Check sheet for the drawn part. Datum: minimum x, y, z corner. Units: mm. A direction names the side the tool comes from. Coordinates: 2 decimals unless noted, no trailing zeros. Loops run counter-clockwise (first coordinate to the right, second up) from the corner with the lowest first, then second, coordinate; pieces in that order, holes last. Notation, with made-up numbers: (84, 4) - (118, 4) arc R8 cw to (118, 12) - close; hole circle Ø8 at (-2.75, -15). An arc over 180 degrees is marked (long way). Answer as CSV lines item,"result". Start each with the question number.
1. Material ranges on line 1 (Y direction, x = 7.5, z = 1); line 2 (X direction, y = 7, z = 1); line 3 (Z direction, x = 5.5, y = 33), recorded low to high. Write a range as [from, to].
2. Cross-section at C-C (z = 22.5). Enter the section's corners in (x, y).
3. Set-up check for the marked faces 1 and 2: record each of +Z, -Z, +X, -X, +Y, -Y from which the full face is reachable in a straight line by a thin tool's end or side.
4. Cross-section at A-A (x = 31.5). Enter the section's corners in (y, z).
5. Release check for a two-part mould opening along X. For the marked faces 3 and 4 record: pulls with the +X half, pulls with the -X half, needs draft (parallel to the pull), parting line crosses it, or undercut.
6. Gauge pin test, flat ends, axial feed: P1, Ø3, axis at y = 10.5, z = 35.5, coming from the +X side (1 decimal); P2, Ø12, axis at x = 48, z = 53.5, coming from the +Y side; P3, Ø6.5, axis at x = 7.5, y = 55.5, coming from the +Z side. Record the tip position at first contact, or that the pin passes through.
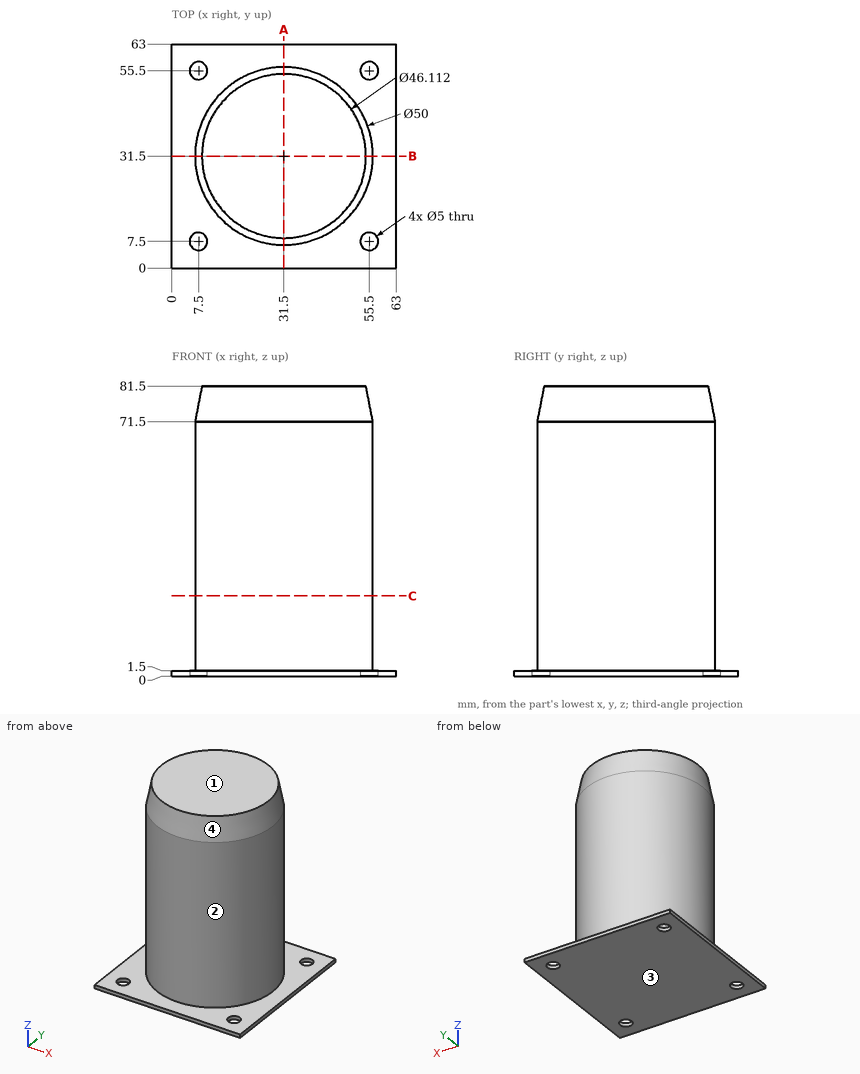
Values follow:
1,line 1,"y = [0, 5], [10, 53], [58, 63]"
1,line 2,"x = [0, 5.05], [9.95, 53.05], [57.95, 63]"
1,line 3,"z = [0, 1.5]"
2,outline,"circle Ø50 at (31.5, 31.5)"
3,face 1,"+Z, +X, -X, +Y, -Y"
3,face 2,"+Z"
4,outline,"(0, 0) - (63, 0) - (63, 1.5) - (56.5, 1.5) - (56.5, 71.5) - (54.56, 81.5) - (8.44, 81.5) - (6.5, 71.5) - (6.5, 1.5) - (0, 1.5) - close"
5,face 3,"needs draft"
5,face 4,"parting line crosses it"
6,P1,"stops at x = 47.1"
6,P2,"stops at y = 54.19"
6,P3,"stops at z = 1.5"
